Design review of the part built by this model. Coordinates are the model's own, in mm. Coordinates: 2 decimals unless noted, no trailing zeros. Write each loop counter-clockwise with the first axis right and the second up, starting at its lowest first coordinate (ties: lowest second). Pieces come first, ordered by that corner, then holes. Notation, with made-up numbers: (-7, 70.5) -> (16, 70.5) arc R9 ccw to (16, 80.5) -> close; hole circle Ø6 at (85.5, 63.25). An arc over 180 degrees is marked (long way). One line per question, with ' | ' between items. Start each with the question number.
Q1. Add section A-A on x = -4. State the section outline as (y, z) points, and give its area (3 significant figures).
Q2. Wall thickness on probe 1 along Y at (x, z) = (-36.5, 0.2); probe 2 along Y at (x, z) = (39.5, 0.8); probe 3 along Y at (x, z) = (-34.5, 0.8): over which ranges is each line inside the solid? List them lowest first.
Q3. Draft analysis for pull direction Y (two halves, no side actions). For faces 1 (the cylindrical face through (49.77, 20.28, 0.76)), 2 (the cylindrical face through (-37.319, 104.172, 0.74)), 3 (the flat face through (-17, 66, 1.5)), state which applies: pulls with the +Y half, pulls with the -Y half, needs draft (parallel to the pull), parting line crosses it, or undercut.
Q4. Add section B-B on y = 68. Give the number of separate pieces and of enclosed holes in the cut face, and give its area (3 significant figures).
Q5. Add section C-C on x = -35.5. State the section outline as (y, z) points, and give its area (3 significant figures).
from build123d import *

# Parameters (mm, degrees)
F0_W     = 93
F0_H     = 93
F0_R     = 2.75
F0_W_2   = 2
F0_H_2   = 73
F1_DEPTH = 1.5
F2_R     = 5


with BuildPart() as f1:
    # F0 (on Top) → F1 (new body)
    with BuildSketch(Plane.XY):
        with Locations((4.777365, 65.356966)):
            Rectangle(F0_W, F0_H)
        with Locations((-36.722635, 23.856966)):
            Circle(F0_R, mode=Mode.SUBTRACT)
        with Locations((46.277365, 23.856966)):
            Circle(F0_R, mode=Mode.SUBTRACT)
        Polygon((-31.722635, 28.856966), (-31.722635, 101.856966), (-26.222635, 101.856966), (-24.222635, 101.856966), (-17.599812, 101.856966), (-15.599812, 101.856966), (-8.976989, 101.856966), (-6.976989, 101.856966), (-0.354166, 101.856966), (1.645834, 101.856966), (8.268656, 101.856966), (10.268656, 101.856966), (16.891479, 101.856966), (18.891479, 101.856966), (25.514302, 101.856966), (27.514302, 101.856966), (34.137125, 101.856966), (36.137125, 101.856966), (41.277365, 101.856966), (41.277365, 28.856966), (36.137125, 28.856966), (34.137125, 28.856966), (27.514302, 28.856966), (25.514302, 28.856966), (18.891479, 28.856966), (16.891479, 28.856966), (10.268656, 28.856966), (8.268656, 28.856966), (1.645834, 28.856966), (-0.354166, 28.856966), (-6.976989, 28.856966), (-8.976989, 28.856966), (-15.599812, 28.856966), (-17.599812, 28.856966), (-24.222635, 28.856966), (-26.222635, 28.856966), align=None, mode=Mode.SUBTRACT)
        with Locations((-36.722635, 106.856966)):
            Circle(F0_R, mode=Mode.SUBTRACT)
        with Locations((46.277365, 106.856966)):
            Circle(F0_R, mode=Mode.SUBTRACT)
        with Locations((-25.222635, 65.356966)):
            Rectangle(F0_W_2, F0_H_2)
        with Locations((-16.599812, 65.356966)):
            Rectangle(F0_W_2, F0_H_2)
        with Locations((-7.976989, 65.356966)):
            Rectangle(F0_W_2, F0_H_2)
        with Locations((0.645834, 65.356966)):
            Rectangle(F0_W_2, F0_H_2)
        with Locations((9.268656, 65.356966)):
            Rectangle(F0_W_2, F0_H_2)
        with Locations((17.891479, 65.356966)):
            Rectangle(F0_W_2, F0_H_2)
        with Locations((26.514302, 65.356966)):
            Rectangle(F0_W_2, F0_H_2)
        with Locations((35.137125, 65.356966)):
            Rectangle(F0_W_2, F0_H_2)
    extrude(amount=F1_DEPTH)

    # F2
    f2_edges = [f1.edges().sort_by_distance(p)[0] for p in [
        (-41.722635, 111.856966, 0.75),
        (51.277365, 111.856966, 0.75),
        (51.277365, 18.856966, 0.75),
        (-41.722635, 18.856966, 0.75),
    ]]
    fillet(f2_edges, radius=F2_R)


solid = f1.part
Output values:
1) outline: (18.86, 0) -> (28.86, 0) -> (28.86, 1.5) -> (18.86, 1.5) -> close; (101.86, 0) -> (111.86, 0) -> (111.86, 1.5) -> (101.86, 1.5) -> close | area: 30.0 mm2
2) probe 1: y = 18.86 to 21.12, 26.6 to 104.12, 109.6 to 111.86 | probe 2: y = 18.86 to 28.86, 101.86 to 111.86 | probe 3: y = 18.86 to 22.24, 25.48 to 105.24, 108.48 to 111.86
3) face 1: pulls with the -Y half | face 2: undercut | face 3: needs draft
4) separate pieces: 10 | enclosed holes: 0 | area: 54.0 mm2
5) outline: (18.86, 0) -> (21.39, 0) -> (21.39, 1.5) -> (18.86, 1.5) -> close; (26.32, 0) -> (104.39, 0) -> (104.39, 1.5) -> (26.32, 1.5) -> close; (109.32, 0) -> (111.86, 0) -> (111.86, 1.5) -> (109.32, 1.5) -> close | area: 125 mm2
